Autodesk Inventor part; units mm, degrees
ref_plane "YZ Plane" through (0, 0, 0) normal (1, 0, 0) x (0, 1, 0)
ref_plane "XZ Plane" through (0, 0, 0) normal (0, 1, 0) x (-1, 0, 0)
ref_plane "XY Plane" through (0, 0, 0) normal (0, 0, 1) x (1, 0, 0)
sketch "Sketch1" plane through (0, 0, 0) normal (0, 1, 0) x (-1, 0, 0)
  circle A0 centre (0, 0) radius 6.35
  line L0 (0, -9.2376) -> (-8, -4.6188)
  line L1 (-8, -4.6188) -> (-8, 4.6188)
  line L2 (-8, 4.6188) -> (0, 9.2376)
  line L3 (0, 9.2376) -> (8, 4.6188)
  line L4 (8, 4.6188) -> (8, -4.6188)
  line L5 (8, -4.6188) -> (0, -9.2376)
  dimension "d0" = 12.7
  dimension "d3" = 16
extrude "Extrusion1" add sketch "Sketch1" along normal mid plane 1050 contours A0 | L0 L1 L2 L3 L4 L5
properties part number "varilla"
For this review, take the finished solid that the model builds, in its own axes (mm). Give positions to 0.01 mm unless a question says otherwise; leave off trailing zeros. Write each loop counter-clockwise with the first axis right and the second up, starting at its lowest first coordinate (ties: lowest second). Pieces come first, ordered by that corner, then holes. Notation, with made-up numbers: M -31.5,58.25 L 1.5,58.25 A35 cw 1.5,96.25 Z; hole C 74,-32 d10. An arc over 180 degrees is marked long. Answer as CSV lines item,"result".
1. Wall thickness on line 1 (Z direction, x = -2.5, y = -440); line 2 (Z direction, x = -0.25, y = 208); line 3 (X direction, y = -157, z = 6.25): over which ranges is each line inside the solid? List them lowest first.
Findings:
line 1,"z = -7.79 to 7.79"
line 2,"z = -9.09 to 9.09"
line 3,"x = -5.17 to 5.17"
2. For pin 1 (1.5 mm diameter, centred on y = 248.5, z = 6.5, fed in from +X); pin 2 (3 mm diameter, centred on x = 4, y = -143.5, fed in from +Z); pin 3 (4 mm diameter, centred on x = -6, y = -77.5, fed in from -Z), all flat-tipped, find the tip position at first contact; note any pin that passes through.
Findings:
pin 1,"stops at x = 6.04"
pin 2,"stops at z = 7.79"
pin 3,"stops at z = -6.93"
3. Consider section A-A, the plane y = 224. Write out the cut boundary in (x, z), then the cut area to 3 significant figures.
Findings:
outline,"M -8,-4.62 L 0,-9.24 L 8,-4.62 L 8,4.62 L 0,9.24 L -8,4.62 Z"
area,"222 mm2"
4. Consider section B-B, the plane x = 3.5. Write out the cut boundary in (y, z), then the cut area to 3 significant figures.
Findings:
outline,"M -525,-7.22 L 525,-7.22 L 525,7.22 L -525,7.22 Z"
area,"15,200 mm2"
